Autodesk Inventor part; units mm, degrees
ref_plane "YZ Plane" through (0, 0, 0) normal (1, 0, 0) x (0, 1, 0)
ref_plane "XZ Plane" through (0, 0, 0) normal (0, 1, 0) x (-1, 0, 0)
ref_plane "XY Plane" through (0, 0, 0) normal (0, 0, 1) x (1, 0, 0)
sketch "Sketch1" plane through (0, 0, 0) normal (0, 0, 1) x (1, 0, 0)
  line L0 (0, 0) -> (70, 0)
  line L1 (70, 0) -> (70, -130)
  line L2 (70, -130) -> (0, -130)
  line L3 (0, -130) -> (0, 0)
  line L4 (0, -10) -> (20, -10)
  line L5 (20, -10) -> (20, -40)
  line L6 (20, -40) -> (0, -40)
  line L7 (0, -40) -> (0, -10)
  line L8 (50, -10) -> (70, -10)
  line L9 (70, -10) -> (70, -40)
  line L10 (70, -40) -> (50, -40)
  line L11 (50, -40) -> (50, -10)
  line L12 (0, -50) -> (20, -50)
  line L13 (20, -50) -> (20, -80)
  line L14 (20, -80) -> (0, -80)
  line L15 (0, -80) -> (0, -50)
  line L16 (50, -50) -> (70, -50)
  line L17 (70, -50) -> (70, -80)
  line L18 (70, -80) -> (50, -80)
  line L19 (50, -80) -> (50, -50)
  line L20 (0, -90) -> (20, -90)
  line L21 (20, -90) -> (20, -120)
  line L22 (20, -120) -> (0, -120)
  line L23 (0, -120) -> (0, -90)
  line L24 (50, -90) -> (70, -90)
  line L25 (70, -90) -> (70, -120)
  line L26 (70, -120) -> (50, -120)
  line L27 (50, -120) -> (50, -90)
  dimension "d0" = 70
  dimension "d1" = 130
  dimension "d2" = 20
  dimension "d3" = 30
  dimension "d4" = 20
  dimension "d5" = 30
  dimension "d6" = 20
  dimension "d7" = 30
  dimension "d8" = 20
  dimension "d9" = 30
  dimension "d10" = 20
  dimension "d11" = 30
  dimension "d12" = 20
  dimension "d13" = 30
  dimension "d14" = 10
  dimension "d15" = 10
  dimension "d16" = 10
  dimension "d17" = 10
  dimension "d18" = 10
  dimension "d19" = 0
  dimension "d20" = 30
extrude "Extrusion1" add sketch "Sketch1" along normal blind 3 contours L0 L1 L8 L11 L10 L16 L19 L18 L24 L27 L26 L2 L3 L22 L21 L20 L14 L13 L12 L6 L5 L4
sketch "Sketch6" plane through (0, 0, 0) normal (0, 0, -1) x (-1, 0, 0)
  line L0 (-50, -10) -> (-70, -10)
  line L1 (-70, -10) -> (-70, -40)
  line L2 (-70, -40) -> (-50, -40)
  line L3 (-50, -40) -> (-50, -10)
  line L4 (-20, -10) -> (0, -10)
  line L5 (0, -10) -> (0, -40)
  line L6 (0, -40) -> (-20, -40)
  line L7 (-20, -40) -> (-20, -10)
  line L8 (-20, -50) -> (0, -50)
  line L9 (0, -50) -> (0, -80)
  line L10 (0, -80) -> (-20, -80)
  line L11 (-20, -80) -> (-20, -50)
  line L12 (0, -90) -> (-20, -90)
  line L13 (-20, -90) -> (-20, -120)
  line L14 (-20, -120) -> (0, -120)
  line L15 (0, -120) -> (0, -90)
  line L16 (-50, -90) -> (-70, -90)
  line L17 (-70, -90) -> (-70, -120)
  line L18 (-70, -120) -> (-50, -120)
  line L19 (-50, -120) -> (-50, -90)
  line L20 (-70, -80) -> (-50, -80)
  line L21 (-50, -80) -> (-50, -50)
  line L22 (-50, -50) -> (-70, -50)
  line L23 (-70, -50) -> (-70, -80)
  point P0 (0, 0)
extrude "Extrusion3" add sketch "Sketch6" against normal blind 8
sketch "Sketch7" plane through (0, 0, 8) normal (0, 0, 1) x (1, 0, 0)
  point P0 (0, 0)
sketch "Sketch8" plane through (0, 0, 8) normal (0, 0, 1) x (1, 0, 0)
  circle A0 centre (10, -25) radius 2.6
  circle A1 centre (28, -25) radius 2.6
  circle A2 centre (42, -25) radius 2.6
  circle A3 centre (60, -25) radius 2.6
  circle A4 centre (10, -65) radius 2.6
  circle A5 centre (28, -65) radius 2.6
  circle A6 centre (42, -65) radius 2.6
  circle A7 centre (59, -65) radius 2.6
  circle A8 centre (11, -105) radius 2.6
  circle A9 centre (28, -105) radius 2.6
  circle A10 centre (42, -105) radius 2.6
  circle A11 centre (60, -105) radius 2.6
  line L0 (20, -10) -> (0, -10)
  line L1 (20, -40) -> (20, -10)
  line L2 (50, -10) -> (50, -40)
  line L3 (70, -10) -> (50, -10)
  line L4 (70, -40) -> (70, -10)
  line L5 (20, -50) -> (0, -50)
  line L6 (20, -90) -> (0, -90)
  line L7 (50, -50) -> (50, -80)
  point P0 (0, 0)
  dimension "d29" = 5.2
  dimension "d30" = 5.2
  dimension "d31" = 5.2
  dimension "d32" = 5.2
  dimension "d33" = 5.2
  dimension "d34" = 5.2
  dimension "d35" = 5.2
  dimension "d36" = 5.2
  dimension "d37" = 5.2
  dimension "d38" = 5.2
  dimension "d39" = 5.2
  dimension "d40" = 5.2
  dimension "d41" = 15
  dimension "d42" = 10
  dimension "d43" = 8
  dimension "d44" = 8
  dimension "d45" = 15
  dimension "d46" = 10
  dimension "d47" = 15
  dimension "d48" = 15
  dimension "d49" = 8
extrude "Extrusion4" cut sketch "Sketch8" against normal through all
properties part number "parking lot frame"
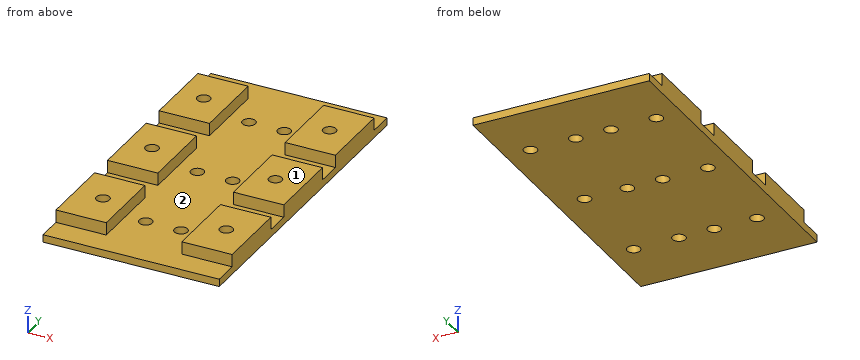
Model file for the job. Use its own axes, mm. Face numbers are marked on the shaded views. Give positions to 0.01 mm unless a question says otherwise; leave off trailing zeros. Write each loop counter-clockwise with the first axis right and the second up, starting at its lowest first coordinate (ties: lowest second). Pieces come first, ordered by that corner, then holes. Notation, with made-up numbers: (43.5, -20) -> (98.5, -20) arc R26 ccw to (98.5, 16) -> close; hole circle Ø6 at (66.5, 66). An arc over 180 degrees is marked (long way). Write item = value, one per line.
(1) Flat gauge pins, fed straight in: P1, Ø2.5, axis at x = 56.5, z = 6.5, coming from the +Y side; P2, Ø8, axis at x = 40.5, y = -101, coming from the +Z side; P3, Ø4, axis at x = 58, z = 6, coming from the -Y side. Where does each tip first touch, or does it go through?
Determined:
P1 = -10
P2 = 3
P3 = -120
(2) Slice it at A-A, the plane x = 60. Give the cut face in (y, z).
Determined:
outline = (-130, 0) -> (-107.6, 0) -> (-107.6, 8) -> (-120, 8) -> (-120, 3) -> (-130, 3) -> close; (-102.4, 0) -> (-67.4, 0) -> (-67.4, 8) -> (-80, 8) -> (-80, 3) -> (-90, 3) -> (-90, 8) -> (-102.4, 8) -> close; (-62.6, 0) -> (-27.6, 0) -> (-27.6, 8) -> (-40, 8) -> (-40, 3) -> (-50, 3) -> (-50, 8) -> (-62.6, 8) -> close; (-22.4, 0) -> (0, 0) -> (0, 3) -> (-10, 3) -> (-10, 8) -> (-22.4, 8) -> close
(3) Mould opens along X. For the marked faces 1 and 2 say: released by +X, released by -X, zero draft, split by the parting line, or undercut.
Determined:
face_1 = zero draft
face_2 = undercut
(4) Slice it at C-C, the plane z = 5.5. Give the number of separate pieces and of enclosed holes in the cut face, then the cut area to 3 significant figures.
Determined:
separate_pieces = 6
enclosed_holes = 6
area = 3,470 mm2
(5) Slice it at B-B, the plane y = -25. Give the cut face in (x, z).
Determined:
outline = (0, 0) -> (7.4, 0) -> (7.4, 8) -> (0, 8) -> close; (12.6, 0) -> (25.4, 0) -> (25.4, 3) -> (20, 3) -> (20, 8) -> (12.6, 8) -> close; (30.6, 0) -> (39.4, 0) -> (39.4, 3) -> (30.6, 3) -> close; (44.6, 0) -> (57.4, 0) -> (57.4, 8) -> (50, 8) -> (50, 3) -> (44.6, 3) -> close; (62.6, 0) -> (70, 0) -> (70, 8) -> (62.6, 8) -> close
(6) Slice it at D-D, the plane y = -92. Give the cut face in (x, z).
Determined:
outline = (0, 0) -> (70, 0) -> (70, 8) -> (50, 8) -> (50, 3) -> (20, 3) -> (20, 8) -> (0, 8) -> close
(7) Probe line 1 along Y through (x, z) = (64, 5.25); line 2 along X through (y, z) = (-14, 5.25); line 3 along Y through (x, z) = (28, 1.9). List the from-to ranges inside material, lowest first.
Determined:
line_1 = -120 to -90, -80 to -50, -40 to -10
line_2 = 0 to 20, 50 to 70
line_3 = -130 to -107.6, -102.4 to -67.6, -62.4 to -27.6, -22.4 to 0
